Work out the finished part from the listing and answer in its coordinate system (mm). A direction names the side the tool comes from. Coordinates: 2 decimals unless noted, no trailing zeros. Write each loop counter-clockwise with the first axis right and the second up, starting at its lowest first coordinate (ties: lowest second). Pieces come first, ordered by that corner, then holes. Notation, with made-up numbers: (61, -1.5) - (70, -1.5) arc R4 ccw to (70, 4.5) - close; hole circle Ø11 at (72, -26.5). An arc over 180 degrees is marked (long way). Use one line per item in the form item = value. Start each with the question number.
Item 1: A cutting plane is placed at A-A (y = 45). Write down the section's boundary in (x, z), then the cut area to 3 significant figures.
Item 2: A cutting plane is placed at B-B (x = 85). Write down the section's boundary in (y, z).
Item 3: A cutting plane is placed at C-C (z = 5). Write down the section's boundary in (x, y), then the cut area to 3 significant figures.
Item 4: For faces 5 (the flat face through (85, 30, 8)), 6 (the flat face through (60, 50, 8)), 7 (the flat face through (100, 85, 8)), 8 (the flat face through (0, 85, 8)), 9 (the flat face through (15, 70, 8)), determine the directions among +Z, -Z, +X, -X, +Y, -Y from which every point of the face is accessible in a straight line to the end or side of a thin tool.
Item 5: A cutting plane is placed at D-D (y = 15). Write down the section's boundary in (x, z), then the cut area to 3 significant figures.
Item 6: Determine the mould class of faces 1 (the flat face through (20, 50, 8)), 2 (the cylindrical face through (20.723, 13.198, 7.888)), 3 (the flat face through (85, 70, 8)), 4 (the flat face through (50, 60, 8)) for opening direction X: released by +X, released by -X, zero draft, split by the parting line, or undercut.
Item 7: Consider probe 1 along Y at (x, z) = (85, 6); probe 2 along X at (y, z) = (44, 8.75); probe 3 along Y at (x, z) = (14, 14). Determine where each line is inside the solid, lowest interval first.
Item 8: Given pin 1 (8 mm diameter, centred on x = 49, z = 4.5, fed in from -Y); pin 2 (5 mm diameter, centred on y = 49.5, z = 10, fed in from +X); pin 3 (4 mm diameter, centred on y = 48.5, z = 3, fed in from -X), each flat-ended and moving along its own axis, determine where each tip first touches the part or whether it passes through.
Autodesk Inventor part; units mm, degrees
ref_plane "YZ Plane" through (0, 0, 0) normal (1, 0, 0) x (0, 1, 0)
ref_plane "XZ Plane" through (0, 0, 0) normal (0, 1, 0) x (-1, 0, 0)
ref_plane "XY Plane" through (0, 0, 0) normal (0, 0, 1) x (1, 0, 0)
sketch "Sketch1" plane through (0, 0, 0) normal (0, 0, 1) x (1, 0, 0)
  line L0 (10, 0) -> (90, 0)
  line L1 (100, 10) -> (100, 20)
  line L2 (90, 30) -> (80, 30)
  line L3 (80, 30) -> (80, 70)
  line L4 (80, 70) -> (90, 70)
  line L5 (100, 80) -> (100, 90)
  line L6 (90, 100) -> (10, 100)
  line L7 (0, 90) -> (0, 80)
  line L8 (10, 70) -> (20, 70)
  line L9 (20, 70) -> (20, 30)
  line L10 (20, 30) -> (10, 30)
  line L11 (0, 10) -> (0, 20)
  line L12 (40, 40) -> (60, 40)
  line L13 (60, 40) -> (60, 60)
  line L14 (60, 60) -> (40, 60)
  line L15 (40, 60) -> (40, 40)
  circle A0 centre (15, 15) radius 6
  circle A1 centre (85, 15) radius 6
  circle A2 centre (15, 85) radius 6
  circle A3 centre (85, 85) radius 6
  arc A4 (10, 100) -> (0, 90) centre (10, 90) ccw
  arc A5 (0, 80) -> (10, 70) centre (10, 80) ccw
  arc A6 (90, 70) -> (100, 80) centre (90, 80) ccw
  arc A7 (100, 90) -> (90, 100) centre (90, 90) ccw
  arc A8 (100, 20) -> (90, 30) centre (90, 20) ccw
  arc A9 (90, 0) -> (100, 10) centre (90, 10) ccw
  arc A10 (0, 10) -> (10, 0) centre (10, 10) ccw
  arc A11 (10, 30) -> (0, 20) centre (10, 20) ccw
  point P0 (0, 0)
  point P1 (100, 70)
  point P2 (100, 100)
  point P3 (0, 70)
  point P4 (0, 30)
  dimension "d0" = 10
extrude "Extrusion1" add sketch "Sketch1" along normal blind 16
properties part number "P2-8"
Answer:
q1.outline = (20, 0) - (40, 0) - (40, 16) - (20, 16) - close; (60, 0) - (80, 0) - (80, 16) - (60, 16) - close
q1.area = 640 mm²
q2.outline = (0, 0) - (9, 0) - (9, 16) - (0, 16) - close; (21, 0) - (30, 0) - (30, 16) - (21, 16) - close; (70, 0) - (79, 0) - (79, 16) - (70, 16) - close; (91, 0) - (100, 0) - (100, 16) - (91, 16) - close
q3.outline = (0, 10) arc R10 ccw to (10, 0) - (90, 0) arc R10 ccw to (100, 10) - (100, 20) arc R10 ccw to (90, 30) - (80, 30) - (80, 70) - (90, 70) arc R10 ccw to (100, 80) - (100, 90) arc R10 ccw to (90, 100) - (10, 100) arc R10 ccw to (0, 90) - (0, 80) arc R10 ccw to (10, 70) - (20, 70) - (20, 30) - (10, 30) arc R10 ccw to (0, 20) - close; hole circle Ø12 at (15, 15); hole circle Ø12 at (15, 85); hole (40, 40) - (60, 40) - (60, 60) - (40, 60) - close; hole circle Ø12 at (85, 15); hole circle Ø12 at (85, 85)
q3.area = 7,380 mm²
q4.face_5 = +Z, -Z, +X
q4.face_6 = +Z, -Z
q4.face_7 = +Z, -Z, +X, +Y, -Y
q4.face_8 = +Z, -Z, -X, +Y, -Y
q4.face_9 = +Z, -Z, -X
q5.outline = (0, 0) - (9, 0) - (9, 16) - (0, 16) - close; (21, 0) - (79, 0) - (79, 16) - (21, 16) - close; (91, 0) - (100, 0) - (100, 16) - (91, 16) - close
q5.area = 1,220 mm²
q6.face_1 = released by -X
q6.face_2 = undercut
q6.face_3 = zero draft
q6.face_4 = undercut
q7.probe_1 = 0 to 9, 21 to 30, 70 to 79, 91 to 100
q7.probe_2 = 20 to 40, 60 to 80
q7.probe_3 = 0 to 9.08, 20.92 to 30, 70 to 79.08, 90.92 to 100
q8.pin_1 = 0
q8.pin_2 = 80
q8.pin_3 = 20
